The model under review builds one solid part; all positions refer to its coordinate system, in mm. Face numbers are marked on the shaded views. A direction names the side the tool comes from. Round coordinates to 2 decimals unless told otherwise and drop trailing zeros. Order: outer loops, then holes, each group sorted by start corner. A loop starts at its lowest first (then second) coordinate and runs counter-clockwise, first axis right, second up.
1) Consider section C-C (x = 112). Give the boundary of the cut face in (y, z).
2) Machinability: for the marked faces 4 and 5, which of the approach directions +Z, -Z, +X, -X, +Y, -Y give a long, thin tool a straight path to every point of the face, cutting with its end or side? Answer none if there is none.
3) Consider section B-B (y = -94.5). Give the boundary of the cut face in (x, z).
4) Clearance check with flat-ended pins moving along their axes: P1, Ø12, axis at x = -104.5, y = -3, coming from the +Z side; P2, Ø6, axis at x = -45.5, z = 168, coming from the +Y side; P3, Ø1.5, axis at x = -22, y = -12, coming from the -Z side; P4, Ø17, axis at y = 56.96, z = 93.52, coming from the +X side. State where each tip first meets the part, or that it passes through.
5) Consider section A-A (z = 268.5). Give the boundary of the cut face in (x, y), then the cut area to 3 significant figures.
6) Mouldability with a two-part tool opening along Y and no side actions: class the marked faces 1, 2 and 3 as pulls with the +Y half, pulls with the -Y half, needs draft (parallel to the pull), parting line crosses it, or undercut.
7) To check wall thickness, follow L1, parallel to X at y = -41.5, z = 89; L2, parallel to Y at x = 95, z = 86.5; L3, parallel to Y at x = -72, z = -5. State the ranges of each line that lie inside material, in increasing order.
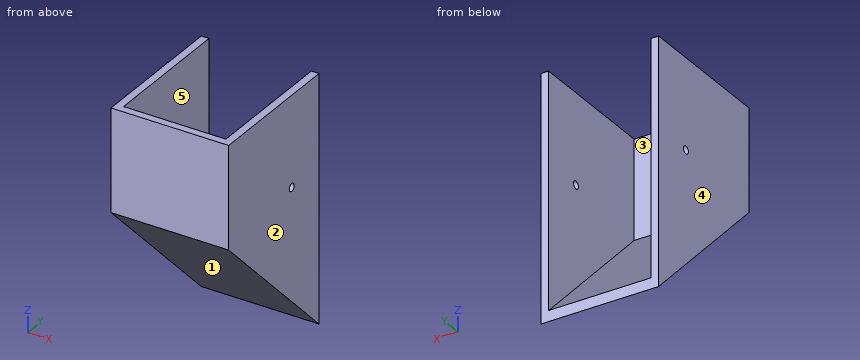
from build123d import *

# Parameters (mm, degrees)
SKETCH2_W           = 292.1
SKETCH2_H           = 635
BOSS_EXTRUDE1_DEPTH = 190.5
CUT_EXTRUDE2_DEPTH  = 381
SHELL1_T            = -19.05
SKETCH5_W           = 292.1
SKETCH5_H           = 635
CUT_EXTRUDE3_DEPTH  = 24.892
SKETCH6_R           = 9.525
CUT_EXTRUDE4_DEPTH  = 514.096
SKETCH10_W          = 292.1
SKETCH10_H          = 610.108
CUT_EXTRUDE7_DEPTH  = 1.693333333


with BuildPart() as part:
    # Sketch2 → Boss-Extrude1 (new body, symmetric)
    with BuildSketch(Plane(origin=(0, 0, 0), x_dir=(1, 0, 0), z_dir=(0, 1, 0))):
        Rectangle(SKETCH2_W, SKETCH2_H)
    extrude(amount=BOSS_EXTRUDE1_DEPTH, both=True)

    # Sketch4 → Cut-Extrude2 (cut)
    with BuildSketch(Plane.ZY.offset(146.05)):
        Polygon((-317.5, 190.5), (63.5, -190.5), (-317.5, -190.5), align=None)
    extrude(amount=-CUT_EXTRUDE2_DEPTH, mode=Mode.SUBTRACT)

    # Shell1
    shell1_openings = [part.faces().sort_by_distance(p)[0] for p in [
        (0, 0, 317.5),
    ]]
    offset(amount=SHELL1_T, openings=shell1_openings, kind=Kind.INTERSECTION)

    # Sketch5 → Cut-Extrude3 (cut)
    with BuildSketch(Plane(origin=(0, 190.5, 0), x_dir=(1, 0, 0), z_dir=(0, 1, 0))):
        Rectangle(SKETCH5_W, SKETCH5_H)
    extrude(amount=-CUT_EXTRUDE3_DEPTH, mode=Mode.SUBTRACT)

    # Sketch6 → Cut-Extrude4 (cut)
    with BuildSketch(Plane.ZY.offset(146.05)):
        with Locations((93.517292524, 56.961208915)):
            Circle(SKETCH6_R)
    extrude(amount=-CUT_EXTRUDE4_DEPTH, mode=Mode.SUBTRACT)

    # Sketch10 → Cut-Extrude7 (cut)
    with BuildSketch(Plane(origin=(0, 165.608, 0), x_dir=(1, 0, 0), z_dir=(0, 1, 0))):
        with Locations((0, -12.446)):
            Rectangle(SKETCH10_W, SKETCH10_H)
    extrude(amount=-CUT_EXTRUDE7_DEPTH, mode=Mode.SUBTRACT)


solid = part.part
Answer below:
1. outline: (-190.5, 63.5) - (163.91, -290.91) - (163.91, -263.97) - (-171.45, 71.39) - (-171.45, 317.5) - (-190.5, 317.5) - close
2. face 4: +Z, -Z, -X, +Y, -Y
2. face 5: +Z, +Y
3. outline: (-146.05, -32.5) - (146.05, -32.5) - (146.05, 317.5) - (127, 317.5) - (127, -5.56) - (-127, -5.56) - (-127, 317.5) - (-146.05, 317.5) - close
4. P1: stops at z = -91.06
4. P2: stops at y = -171.45
4. P3: stops at z = -115.75
4. P4: passes through
5. outline: (-146.05, -190.5) - (146.05, -190.5) - (146.05, 163.91) - (127, 163.91) - (127, -171.45) - (-127, -171.45) - (-127, 163.91) - (-146.05, 163.91) - close
5. area: 18,300 mm2
6. face 1: pulls with the -Y half
6. face 2: needs draft
6. face 3: pulls with the +Y half
7. L1: x = -146.05 to -127, 127 to 146.05
7. L2: y = -190.5 to -171.45
7. L3: y = -122 to -95.06
